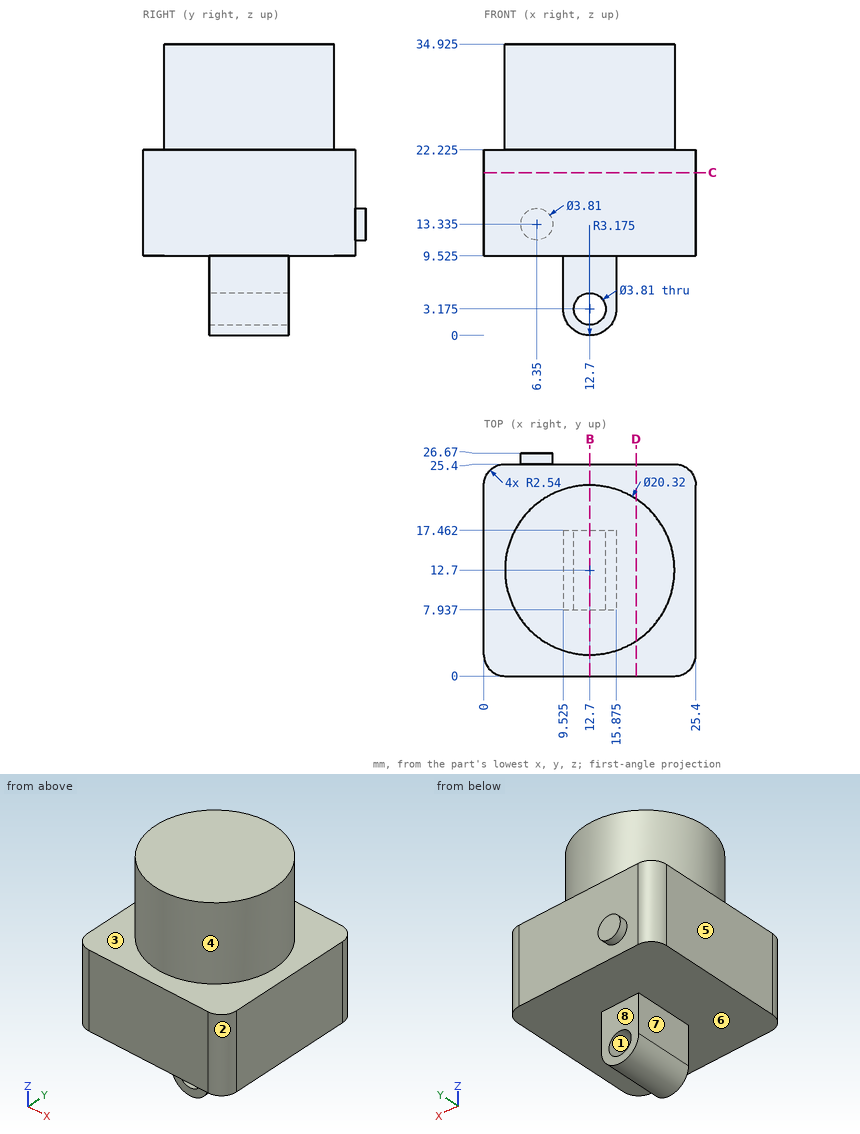
For this review, use the dimensioned drawing (mm, ordinates from the lowest corner) and the shaded views. A direction names the side the tool comes from. Coordinates: 2 decimals unless noted, no trailing zeros. Loops run counter-clockwise (first coordinate to the right, second up) from the corner with the lowest first, then second, coordinate; pieces in that order, holes last. Notation, with made-up numbers: (49.25, -15.75) -> (68.25, -15.75) arc R27 ccw to (68.25, 12.25) -> close; hole circle Ø4 at (37, 5.25). An arc over 180 degrees is marked (long way). Return JSON: item names as keys, results as strings. Group by question number.
(1) For pin 1 Ø3 at (x, z) = (12.5, 6.5) entering from +Y; pin 2 Ø5 at (x, z) = (12.5, 6) entering from -Y; pin 3 Ø4 at (x, y) = (13, 23) entering from -Z (1 decimal), all flat-tipped, find the tip position at first contact; note any pin that passes through.
(2) Tool access review of the marked faces 4, 5, 6, 7 and 8: name each direction out of +Z, -Z, +X, -X, +Y, -Y from which nothing blocks a thin tool from reaching the whole face with its end or side.
(3) Consider section D-D, the plane x = 18.25. Give the boundary of the cut face in (y, z) (1 decimal), plus the area to 3 significant figures.
(4) Mouldability with a two-part tool opening along X and no side actions: class the marked faces 1, 2 and 3 as pulls with the +X half, pulls with the -X half, needs draft (parallel to the pull), parting line crosses it, or undercut.
(5) Consider section B-B, the plane x = 12.7. Give the boundary of the cut face in (y, z) (1 decimal), plus the area to 3 significant figures.
(6) Consider section C-C, the plane z = 19.5. Give the boundary of the cut face in (x, y), plus the area to 3 significant figures.
(7) To check wall thickness, follow L1, parallel to Z at x = 9.25, y = 9.5 (1 decimal); L2, parallel to Y at x = 12.5, z = 12; L3, parallel to Z at x = 17.25, y = 23.75 (1 decimal). State the ranges of each line that lie inside material, in increasing order.
Results below:
{
 "1": {"pin 1": "stops at y = 17.46", "pin 2": "stops at y = 7.94", "pin 3": "stops at z = 9.5"},
 "2": {"face 4": "+Z", "face 5": "+Z, -Z, -X, +Y, -Y", "face 6": "-Z", "face 7": "-Z, -X, +Y, -Y", "face 8": "-Z, +X, -X, +Y"},
 "3": {"outline": "(0, 9.5) -> (25.4, 9.5) -> (25.4, 22.2) -> (21.2, 22.2) -> (21.2, 34.9) -> (4.2, 34.9) -> (4.2, 22.2) -> (0, 22.2) -> close", "area": "539 mm2"},
 "4": {"face 1": "undercut", "face 2": "pulls with the +X half", "face 3": "needs draft"},
 "5": {"outline": "(0, 9.5) -> (7.9, 9.5) -> (7.9, 5.1) -> (17.5, 5.1) -> (17.5, 9.5) -> (25.4, 9.5) -> (25.4, 22.2) -> (22.9, 22.2) -> (22.9, 34.9) -> (2.5, 34.9) -> (2.5, 22.2) -> (0, 22.2) -> close; (7.9, 0) -> (17.5, 0) -> (17.5, 1.3) -> (7.9, 1.3) -> close", "area": "635 mm2"},
 "6": {"outline": "(0, 2.54) arc R2.54 ccw to (2.54, 0) -> (22.86, 0) arc R2.54 ccw to (25.4, 2.54) -> (25.4, 22.86) arc R2.54 ccw to (22.86, 25.4) -> (2.54, 25.4) arc R2.54 ccw to (0, 22.86) -> close", "area": "640 mm2"},
 "7": {"L1": "z = 9.5 to 34.9", "L2": "y = 0 to 25.4", "L3": "z = 9.5 to 22.2"}
}
